Autodesk Inventor part; units mm, degrees
ref_plane "YZ Plane" through (0, 0, 0) normal (1, 0, 0) x (0, 1, 0)
ref_plane "XZ Plane" through (0, 0, 0) normal (0, 1, 0) x (-1, 0, 0)
ref_plane "XY Plane" through (0, 0, 0) normal (0, 0, 1) x (1, 0, 0)
sketch "Sketch36" plane through (0, 0, 0) normal (0, 1, 0) x (-1, 0, 0)
  line L0 (29.1617, 36.148) -> (29.1617, -76.352)
  line L1 (29.1617, -76.352) -> (-44.8383, -76.352)
  line L2 (-44.8383, -76.352) -> (-44.8383, 36.148)
  line L3 (-44.8383, 36.148) -> (29.1617, 36.148)
  point P0 (0, 0)
  dimension "d191" = 112.5
  dimension "d192" = 74
extrude "Extrusion21" add sketch "Sketch36" along normal blind 3
sketch "Sketch37" plane through (0, 3, 0) normal (0, 1, 0) x (1, 0, 0)
  line L0 (-29.1617, 76.352) -> (-29.1617, -36.148)
  line L1 (-29.1617, -36.148) -> (-29.1617, 76.352)
  line L2 (44.8383, -36.148) -> (44.8383, 76.352)
  line L3 (-29.1617, 76.352) -> (44.8383, 76.352)
  line L4 (44.8383, 76.352) -> (44.8383, -36.148)
  line L5 (-29.1617, -36.148) -> (44.8383, -36.148)
  line L6 (44.8383, -36.148) -> (-29.1617, -36.148)
  line L7 (-26.1617, -33.148) -> (41.8383, -33.148)
  line L8 (41.8383, 73.352) -> (-26.1617, 73.352)
  line L9 (-26.1617, 73.352) -> (-26.1617, -33.148)
  line L10 (41.8383, -33.148) -> (41.8383, 40.852)
  line L11 (41.8383, 40.852) -> (44.8383, 40.852)
  line L12 (41.8383, 73.352) -> (41.8383, 64.852)
  line L13 (41.8383, 64.852) -> (44.8383, 64.852)
  point P0 (0, 0)
  point P1 (43.3383, 64.852)
  dimension "d195" = 3
  dimension "d197" = 3
  dimension "d198" = 3
  dimension "d199" = 3
  dimension "d203" = 8.5
  dimension "d261" = 24
extrude "Extrusion22" add sketch "Sketch37" along normal blind 5.5 contours L3 L2 L13 L12 L8 L9 L7 L10 L11 L5 L0
sketch "Sketch39" plane through (0, 0, 0) normal (0, -1, 0) x (1, 0, 0)
  circle A0 centre (8.3383, -20.852) radius 1.4
  line L0 (-29.1617, -76.352) -> (-29.1617, 36.148)
  line L1 (44.8383, 36.148) -> (44.8383, -76.352)
  line L2 (-25.1617, -14.852) -> (-28.1617, -14.852)
  line L3 (-28.1617, -14.852) -> (-28.1617, -23.852)
  line L4 (-28.1617, -23.852) -> (-25.1617, -23.852)
  line L5 (-25.1617, -23.852) -> (-25.1617, -14.852)
  line L6 (-29.1617, 36.148) -> (44.8383, 36.148)
  point P0 (0, 0)
  dimension "d217" = 9
  dimension "d218" = 3
  dimension "d295" = 36.5
  dimension "d296" = 51
extrude "Extrusion25" add sketch "Sketch39" along normal blind 10 contours L5 L4 L3 L2
sketch "Sketch43" plane through (0, 0, 0) normal (0, -1, 0) x (1, 0, 0)
  circle A0 centre (24.8383, -37.352) radius 1
  circle A1 centre (24.8383, -46.352) radius 1
  line L0 (44.8383, -76.352) -> (-29.1617, -76.352)
  circle A2 centre (8.3383, -20.852) radius 1.4
  line L1 (-29.1617, 36.148) -> (44.8383, 36.148)
  line L2 (44.8383, 36.148) -> (44.8383, -76.352)
  point P0 (0, 0)
  dimension "d252" = 2
  dimension "d253" = 2
  dimension "d254" = 9
  dimension "d256" = 30
  dimension "d258" = 20
extrude "Extrusion29" cut sketch "Sketch43" against normal blind 10 contours A0 | A1
sketch "Sketch45" plane through (0, 3, 0) normal (0, 1, 0) x (1, 0, 0)
  line L0 (41.8383, -33.148) -> (41.8383, 40.852)
  line L1 (41.8383, -14.148) -> (-26.1617, -14.148)
  line L2 (-26.1617, 73.352) -> (-26.1617, -33.148)
  line L3 (-26.1617, -24.148) -> (41.8383, -24.148)
  line L4 (41.8383, -24.148) -> (41.8383, -14.148)
  line L5 (41.8383, -33.148) -> (-26.1617, -33.148)
  line L6 (-26.1617, 64.352) -> (42.4383, 64.352)
  line L7 (42.4383, 64.352) -> (42.4383, 54.352)
  line L8 (42.4383, 54.352) -> (-26.1617, 54.352)
  line L9 (-26.1617, 64.352) -> (-26.1617, 54.352)
  line L10 (-26.1617, 73.352) -> (41.8383, 73.352)
  point P0 (0, 0)
  point P1 (41.8383, -24.148)
  dimension "d274" = 10
  dimension "d275" = 9
  dimension "d276" = 9
  dimension "d277" = 10
extrude "Extrusion31" add sketch "Sketch45" along normal blind 3 contours L2 L6 L7 L8 | L3 L2 L1 L0
sketch "Sketch48" plane through (-29.1617, 0, 36.148) normal (-1, 0, 0) x (0, 0, 1)
  circle A0 centre (-55.5, -5) radius 1.75
  line L0 (-51, 0) -> (-51, -10)
  line L1 (-51, -10) -> (-60, -10)
  point P0 (-36.148, 0)
  dimension "d297" = 3.5
  dimension "d298" = 4.5
  dimension "d299" = 5
extrude "Extrusion34" cut sketch "Sketch48" against normal blind 10
sketch "Sketch50" plane through (44.8383, 0, 36.148) normal (1, 0, 0) x (0, 0, -1)
  line L0 (0, 0) -> (0, 8.5)
  line L1 (0, 5.75) -> (1.5, 4.25)
  line L2 (1.5, 4.25) -> (0, 2.75)
  line L3 (0, 8.5) -> (77, 8.5)
  point P0 (36.148, 0)
  dimension "d307" = 4.25
  dimension "d314" = 45
  dimension "d316" = 1.5
extrude "Extrusion36" cut sketch "Sketch50" against normal blind 75
sketch "Sketch51" plane through (44.8383, 0, 36.148) normal (1, 0, 0) x (0, 0, -1)
  line L0 (112.5, 0) -> (112.5, 8.5)
  line L1 (112.5, 5.75) -> (111, 4.25)
  line L2 (111, 4.25) -> (112.5, 2.75)
  line L3 (101, 8.5) -> (112.5, 8.5)
  point P0 (36.148, 0)
  dimension "d317" = 45
  dimension "d318" = 45
  dimension "d319" = 4.25
  dimension "d320" = 1.5
extrude "Extrusion37" cut sketch "Sketch51" against normal blind 75
sketch "Sketch52" plane through (0, 0, 0) normal (0, -1, 0) x (1, 0, 0)
  circle A0 centre (8.3383, -20.852) radius 1.4
  circle A1 centre (8.3383, -20.852) radius 1.4
  point P0 (0, 0)
  dimension "d324" = 2.8
extrude "Extrusion38" add sketch "Sketch52" along normal blind 5
properties part number "plate"
Input: part model. Units: mm. Frame: model coordinates. A direction names the side the tool comes from. Coordinates: 2 decimals unless noted, no trailing zeros. Write each loop counter-clockwise with the first axis right and the second up, starting at its lowest first coordinate (ties: lowest second). Pieces come first, ordered by that corner, then holes. Notation, with made-up numbers: M -1.5,-13 L 39.5,-13 A31 ccw 39.5,18 Z; hole C -25,-21.75 d1. An arc over 180 degrees is marked long. Answer as a JSON object with one key per item and string values. Group by question number.
(1) Set-up query: faces 1 (the face through (9, 4, -54.352)), 2 (the face through (-28.162, -5, -17)), 3 (the face through (41.838, 6, -3)), 4 (the face through (-26.683, -5.67, -17.735)). Return all of +Z, -Z, +X, -X, +Y, -Y with unobstructed straight access to the full face (end or side cutting, diameter ignored); none if empty.
(2) Section D-D on z = -16. Output: boundary loops of the cut face in (x, y), plus the area to 3 significant figures.
(3) Mould query, pull axis X, two halves, no side actions, for faces 5 (the face through (43, 6, -64.852)), 6 (the face through (44.838, 4, -21)), 7 (the face through (10, 3, -29)), 8 (the face through (-29.162, 4, -19)). Classes: pulls with the +X half, pulls with the -X half, needs draft (parallel to the pull), parting line crosses it, or undercut.
(4) Section C-C on z = 4. Output: boundary loops of the cut face in (x, y), plus the area to 3 significant figures.
(5) Contact query for flat-ended pins moving along their axis: P1, Ø5, axis at x = -7.5, z = -6.5, coming from the -Y side; P2, Ø1, axis at x = -9, z = -23.5, coming from the +Y side; P3, Ø1.8, axis at x = 24.84, z = -37.35, coming from the +Y side; P4, Ø2.5, axis at x = -27.5, y = -3, coming from the +Z side. Output: stop coordinate, or through.
(6) Ray query, line 1 along Z through (x, y) = (26.5, 4.25); line 2 along X through (y, z) = (6.25, -33); line 3 along Z through (x, y) = (34.5, 6.5). Return the intervals inside material, ascending. Write a range as [from, to].
(7) Section B-B on x = -3. Output: boundary loops of the cut face in (y, z).
(8) Section A-A on z = -63. Output: boundary loops of the cut face in (x, y).
Result set:
{
 "1": {"face 1": "+X, +Y", "face 2": "+Z, -Z, -X, -Y", "face 3": "+Y", "face 4": "-X"},
 "2": {"outline": "M -29.16,0 L -28.16,0 L -28.16,-10 L -25.16,-10 L -25.16,0 L 44.84,0 L 44.84,8.5 L 41.84,8.5 L 41.84,3 L -26.16,3 L -26.16,8.5 L -29.16,8.5 Z", "area": "285 mm2"},
 "3": {"face 5": "needs draft", "face 6": "pulls with the +X half", "face 7": "undercut", "face 8": "pulls with the -X half"},
 "4": {"outline": "M -29.16,0 L 44.84,0 L 44.84,8.5 L 41.84,8.5 L 41.84,3 L -26.16,3 L -26.16,8.5 L -29.16,8.5 Z", "area": "255 mm2"},
 "5": {"P1": "stops at y = 0", "P2": "stops at y = 3", "P3": "passes through", "P4": "stops at z = -14.85"},
 "6": {"line 1": "z = [-74.85, -73.35], [-64.35, -54.35], [14.15, 24.15], [33.15, 34.65]", "line 2": "x = [-29.16, -26.16], [41.84, 44.84]", "line 3": "z = [-76.35, -73.35], [33.15, 36.15]"},
 "7": {"outline": "M 0,-76.35 L 2.75,-76.35 L 4.25,-74.85 L 5.75,-76.35 L 8.5,-76.35 L 8.5,-73.35 L 3,-73.35 L 3,-64.35 L 6,-64.35 L 6,-54.35 L 3,-54.35 L 3,14.15 L 6,14.15 L 6,24.15 L 3,24.15 L 3,33.15 L 8.5,33.15 L 8.5,36.15 L 5.75,36.15 L 4.25,34.65 L 2.75,36.15 L 0,36.15 Z"},
 "8": {"outline": "M -29.16,0 L 44.84,0 L 44.84,3 L 42.44,3 L 42.44,6 L -26.16,6 L -26.16,8.5 L -29.16,8.5 Z"}
}
